from build123d import *

# Parameters (mm, degrees)
EXTRUDE_1_DEPTH     = 7.5
CUT_EXTRUDE_START   = 10.884514
SKETCH_2_R          = 1.912136214
SKETCH_2_W          = 7.090261775
SKETCH_2_H          = 13.093091483
SKETCH_2_R_2        = 1.380933403
SKETCH_2_R_3        = 0.65
CUT_EXTRUDE_1_DEPTH = 4.5
CUT_EXTRUDE_2_DEPTH = 2
SKETCH_2_6_R        = 0.65
EXTRUDE_3_DEPTH     = 3.7
CUT_EXTRUDE_START_2 = -7.090262
SKETCH_4_R          = 1.411151221
SKETCH_4_R_2        = 0.775543873
CUT_EXTRUDE_3_DEPTH = 1.5
SKETCH_5_W          = 1.46101298
SKETCH_5_H          = 4.936486251
SKETCH_5_R          = 1.912136214
CUT_EXTRUDE_4_DEPTH = 18.867005063
EXTRUDE_START       = 1.643513749
EXTRUDE_4_DEPTH     = 0.92


# Read off the part's stored shape, not the designer's step: Бобышка-Вытянуть4
with BuildPart() as part:
    # Эскиз1 → Бобышка-Вытянуть1 (new, symmetric)
    with BuildSketch(Plane.XY):
        Polygon((-7.090261775, 0), (-7.090261775, 7.678308116), (-0.349095572, 10.884514209), (4.975912264, 10.884514209), (5.725642609, 7.058967063), (6.436925244, 7.058967063), (6.436925244, 0.551631224), (4.538262875, 0), align=None)
    extrude(amount=EXTRUDE_1_DEPTH, both=True)

    # Эскиз2 → Вырез-Вытянуть1 (cut)
    # profile 1 of 7: a face of its own
    with BuildSketch(Plane(origin=(0, 0, 0), x_dir=(1, 0, 0), z_dir=(0, 1, 0)).offset(CUT_EXTRUDE_START)):
        with Locations(Location((2.535525991, 5.024679523, 0), (0, 0, 90))):
            Circle(SKETCH_2_R)
    # profile 2 of 7: a face of its own
    with BuildSketch(Plane(origin=(0, 0, 0), x_dir=(1, 0, 0), z_dir=(0, 1, 0)).offset(CUT_EXTRUDE_START)):
        with Locations(Location((2.535525991, 0, 0), (0, 0, 90))):
            Circle(SKETCH_2_R)
    # profile 3 of 7: a face of its own
    with BuildSketch(Plane(origin=(0, 0, 0), x_dir=(1, 0, 0), z_dir=(0, 1, 0)).offset(CUT_EXTRUDE_START)):
        with Locations(Location((2.535525991, -5.063513749, 0), (0, 0, 90))):
            Circle(SKETCH_2_R)
    # profile 4 of 7: a face of its own
    with BuildSketch(Plane(origin=(0, 0, 0), x_dir=(1, 0, 0), z_dir=(0, 1, 0)).offset(CUT_EXTRUDE_START)):
        with Locations((-3.545130888, 0.03776166)):
            Rectangle(SKETCH_2_W, SKETCH_2_H)
        with Locations((-2.812641214, -5.063513749)):
            Circle(SKETCH_2_R_2, mode=Mode.SUBTRACT)
        with Locations((-2.812641214, 0)):
            Circle(SKETCH_2_R_2, mode=Mode.SUBTRACT)
        with Locations((-2.812641214, 5.024679523)):
            Circle(SKETCH_2_R_2, mode=Mode.SUBTRACT)
    # profile 5 of 7: a face of its own
    with BuildSketch(Plane(origin=(0, 0, 0), x_dir=(1, 0, 0), z_dir=(0, 1, 0)).offset(CUT_EXTRUDE_START)):
        with Locations((-2.812641214, -5.063513749)):
            Circle(SKETCH_2_R_3)
    # profile 6 of 7: a face of its own
    with BuildSketch(Plane(origin=(0, 0, 0), x_dir=(1, 0, 0), z_dir=(0, 1, 0)).offset(CUT_EXTRUDE_START)):
        with Locations((-2.812641214, 0)):
            Circle(SKETCH_2_R_3)
    # profile 7 of 7: a face of its own
    with BuildSketch(Plane(origin=(0, 0, 0), x_dir=(1, 0, 0), z_dir=(0, 1, 0)).offset(CUT_EXTRUDE_START)):
        with Locations((-2.812641214, 5.024679523)):
            Circle(SKETCH_2_R_3)
    extrude(amount=-CUT_EXTRUDE_1_DEPTH, mode=Mode.SUBTRACT)

    # Эскиз3 → Вырез-Вытянуть2 (cut)
    with BuildSketch(Plane(origin=(6.436925244, 0, 0), x_dir=(0, 0, -1), z_dir=(1, 0, 0))):
        with BuildLine():
            Line((1.75, 5.953109404), (-1.75, 5.953109404))
            Line((-1.75, 5.953109404), (-1.75, 2.794090542))
            ThreePointArc((-1.75, 2.794090542), (0, 1.131399682), (1.75, 2.794090542))
            Line((1.75, 2.794090542), (1.75, 5.953109404))
        make_face()
        with BuildLine():
            Line((3.25, 5.953109404), (3.25, 2.794090542))
            ThreePointArc((3.25, 2.794090542), (5, 1.131399682), (6.75, 2.794090542))
            Line((6.75, 2.794090542), (6.75, 5.953109404))
            Line((6.75, 5.953109404), (3.25, 5.953109404))
        make_face()
        with BuildLine():
            Line((-6.75, 5.953109404), (-6.75, 2.794090542))
            ThreePointArc((-6.75, 2.794090542), (-5, 1.131399682), (-3.25, 2.794090542))
            Line((-3.25, 2.794090542), (-3.25, 5.953109404))
            Line((-3.25, 5.953109404), (-6.75, 5.953109404))
        make_face()
    extrude(amount=-CUT_EXTRUDE_2_DEPTH, mode=Mode.SUBTRACT)

    # Эскиз2<6> → Бобышка-Вытянуть3 (add)
    with BuildSketch(Plane(origin=(0, 0, 0), x_dir=(1, 0, 0), z_dir=(0, 1, 0))):
        with Locations((-2.812641214, 5.024679523)):
            Circle(SKETCH_2_6_R)
        with Locations((-2.812641214, 0)):
            Circle(SKETCH_2_6_R)
        with Locations((-2.812641214, -5.063513749)):
            Circle(SKETCH_2_6_R)
    extrude(amount=-EXTRUDE_3_DEPTH)

    # Эскиз4 → Вырез-Вытянуть3 (cut)
    # profile 1 of 7: a face of its own
    with BuildSketch(Plane(origin=(0, 0, 0), x_dir=(0, 0, -1), z_dir=(1, 0, 0)).offset(CUT_EXTRUDE_START_2)):
        with Locations((5.042912497, 4.548641576)):
            Circle(SKETCH_4_R)
        with Locations((5.042912497, 4.548641576)):
            Circle(SKETCH_4_R_2, mode=Mode.SUBTRACT)
    # profile 2 of 7: a face of its own
    with BuildSketch(Plane(origin=(0, 0, 0), x_dir=(0, 0, -1), z_dir=(1, 0, 0)).offset(CUT_EXTRUDE_START_2)):
        with Locations((5.042912497, 4.548641576)):
            Circle(SKETCH_4_R_2)
    # profile 3 of 7: a face of its own
    with BuildSketch(Plane(origin=(0, 0, 0), x_dir=(0, 0, -1), z_dir=(1, 0, 0)).offset(CUT_EXTRUDE_START_2)):
        with Locations((0, 4.548641576)):
            Circle(SKETCH_4_R)
        with Locations((0, 4.548641576)):
            Circle(SKETCH_4_R_2, mode=Mode.SUBTRACT)
    # profile 4 of 7: a face of its own
    with BuildSketch(Plane(origin=(0, 0, 0), x_dir=(0, 0, -1), z_dir=(1, 0, 0)).offset(CUT_EXTRUDE_START_2)):
        with Locations((0, 4.548641576)):
            Circle(SKETCH_4_R_2)
    # profile 5 of 7: a face of its own
    with BuildSketch(Plane(origin=(0, 0, 0), x_dir=(0, 0, -1), z_dir=(1, 0, 0)).offset(CUT_EXTRUDE_START_2)):
        with Locations((-5.053327676, 4.548641576)):
            Circle(SKETCH_4_R)
        with Locations((-5.053327676, 4.548641576)):
            Circle(SKETCH_4_R_2, mode=Mode.SUBTRACT)
    # profile 6 of 7: a face of its own
    with BuildSketch(Plane(origin=(0, 0, 0), x_dir=(0, 0, -1), z_dir=(1, 0, 0)).offset(CUT_EXTRUDE_START_2)):
        with Locations((-5.053327676, 4.548641576)):
            Circle(SKETCH_4_R_2)
    # profile 7 of 7: a face of its own
    with BuildSketch(Plane(origin=(0, 0, 0), x_dir=(0, 0, -1), z_dir=(1, 0, 0)).offset(CUT_EXTRUDE_START_2)):
        Polygon((6.413915436, 2.503175658), (3.026112508, 2.503175658), (3.026112508, 5.869671649), (2.131221168, 5.869671649), (2.131221168, 2.503175658), (0.436105724, 2.500060238), (-1.258778832, 2.528210165), (-1.258778832, 0.951386535), (0.31785264, 0.932735686), (6.413915436, 0.932735686), align=None)
    extrude(amount=CUT_EXTRUDE_3_DEPTH, mode=Mode.SUBTRACT)

    # Эскиз5 → Вырез-Вытянуть4 (cut, through all)
    # profile 1 of 4: a face of its own
    with BuildSketch(Plane(origin=(0, 10.884514209, 0), x_dir=(1, 0, 0), z_dir=(0, 1, 0))):
        Polygon((0, -2.563513749), (-7.090261775, -2.563513749), (-7.090261775, -7.5), (-0.349095572, -7.5), (-0.349095572, -6.508784082), (0, -6.508784082), align=None)
    # profile 2 of 4: a face of its own
    with BuildSketch(Plane(origin=(0, 10.884514209, 0), x_dir=(1, 0, 0), z_dir=(0, 1, 0))):
        with Locations((5.706418754, -5.031756875)):
            Rectangle(SKETCH_5_W, SKETCH_5_H)
    # profile 3 of 4: a face of its own
    with BuildSketch(Plane(origin=(0, 10.884514209, 0), x_dir=(1, 0, 0), z_dir=(0, 1, 0))):
        Polygon((4.975912264, -2.563513749), (0, -2.563513749), (0, -6.508784082), (-0.349095572, -6.508784082), (-0.349095572, -7.5), (4.975912264, -7.5), align=None)
        with Locations((2.535525991, -5.063513749)):
            Circle(SKETCH_5_R, mode=Mode.SUBTRACT)
    # profile 4 of 4: a face of its own
    with BuildSketch(Plane(origin=(0, 10.884514209, 0), x_dir=(1, 0, 0), z_dir=(0, 1, 0))):
        with Locations((2.535525991, -5.063513749)):
            Circle(SKETCH_5_R)
    extrude(amount=-CUT_EXTRUDE_4_DEPTH, mode=Mode.SUBTRACT)

    # Бобышка-Вытянуть4 outline → Бобышка-Вытянуть4 (add)
    with BuildSketch(Plane.XY.offset(EXTRUDE_START)):
        Polygon((-7.090261775, 7.678308116), (-7.090261775, 6.384514209), (0, 6.384514209), (0, 11.050549627), align=None)
    extrude(amount=EXTRUDE_4_DEPTH)


solid = part.part
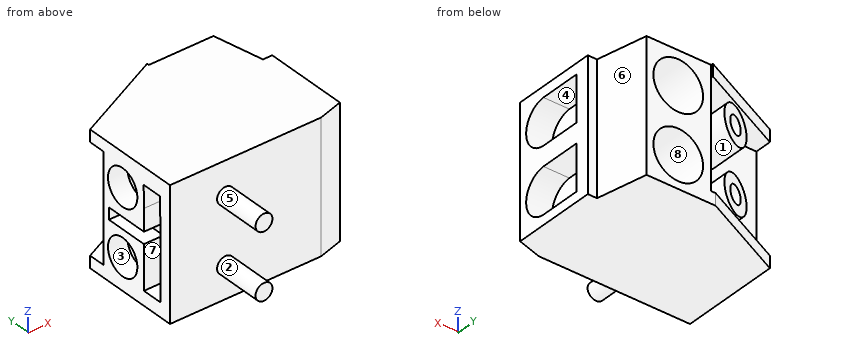
The listing builds one solid part. Answer for the finished solid, in the listing's coordinates (mm). Face numbers are marked on the shaded views. A direction names the side the tool comes from. Round coordinates to 2 decimals unless told otherwise and drop trailing zeros. Order: outer loops, then holes, each group sorted by start corner. A loop starts at its lowest first (then second) coordinate and runs counter-clockwise, first axis right, second up. Notation, with made-up numbers: (60, 43.5) -> (86, 43.5) arc R25 cw to (86, 73.5) -> close; hole circle Ø5 at (66.25, 74). An arc over 180 degrees is marked (long way). Write each question's results on one line, items separated by ' | '. Start each with the question number.
Q1. The mould has two halves that part along X. Classify the marked faces 5, 6, 7 and 8: pulls with the +X half, pulls with the -X half, needs draft (parallel to the pull), parting line crosses it, or undercut.
Q2. Each of these flat-tipped pins is pushed along its axis until it touches: pin 1 (1 mm diameter, centred on x = -3.5, z = -3.5, fed in from -Y); pin 2 (1 mm diameter, centred on x = -2.5, z = 0, fed in from +Y); pin 3 (1 mm diameter, centred on y = 4.5, z = 0.5, fed in from +X). Where does it stop, or does it pass through?
Q3. Which of the six approach directions +Z, -Z, +X, -X, +Y, -Y give full straight-line access (tool end or side, diameter ignored) to the marked faces 1, 2, 3 and 4?
Q4. Straight lines are drawn through the part: probe 1 along Y at (x, z) = (-6.45, 0); probe 2 along Z at (x, y) = (-6, 7.75); probe 3 along Z at (x, y) = (5.75, 3.75). For each, find the intervals that lie inside material, in ascending order. Write a range as from..to.
Q5. Find section A-A (y = 9.75). Determine the outline of the cut face in (x, z), then the cut area to 3 significant figures.
Q6. Find section C-C (x = -5). Determine the outline of the cut face in (y, z).
Worked answers:
1) face 5: parting line crosses it | face 6: pulls with the +X half | face 7: needs draft | face 8: undercut
2) pin 1: stops at y = 0 | pin 2: stops at y = 10.1 | pin 3: stops at x = 4.44
3) face 1: +Y | face 2: -Y | face 3: -X | face 4: +X
4) probe 1: y = 0..0.94, 2.51..3.14, 5.96..6.38 | probe 2: z = -7.5..-6.58, 1.64..2.56 | probe 3: z = -7.5..-6.75, -3.25..-1.75, 1.75..2.56
5) outline: (-2.73, -7.5) -> (5.2, -7.5) -> (5.2, 2.56) -> (-2.73, 2.56) -> (-2.73, 1.64) -> (0, 1.64) -> (0, -6.58) -> (-2.73, -6.58) -> close; (-2.73, -6.4) arc R1.38 ccw to (-2.73, -3.65) -> (-2.73, -4.38) arc R0.65 cw to (-2.73, -5.67) -> close; (-2.73, -1.38) arc R1.38 ccw to (-2.73, 1.38) -> (-2.73, 0.65) arc R0.65 cw to (-2.73, -0.65) -> close; hole circle Ø3.82 at (2.54, -5.02); hole circle Ø3.82 at (2.54, 0) | area: 38.8 mm2
6) outline: (0, -7.5) -> (8.67, -7.5) -> (8.67, -6.58) -> (6.38, -6.58) -> (6.38, 1.64) -> (8.67, 1.64) -> (8.67, 2.56) -> (0, 2.56) -> close
